Could you check a few things on this model? Use its own coordinates, in mm. A direction names the side the tool comes from. Round coordinates to 2 decimals unless told otherwise and drop trailing zeros. Write each loop counter-clockwise with the first axis right and the second up, starting at its lowest first coordinate (ties: lowest second). Pieces come first, ordered by that corner, then holes. Notation, with made-up numbers: (66.5, 25.25) - (124.5, 25.25) arc R9 cw to (124.5, 38.25) - close; hole circle Ø5 at (61.25, 82). An arc over 180 degrees is marked (long way). Write each question's results on one line, items separated by ' | '. Start each with the question number.
(1) For P1, Ø5, axis at y = 44, z = 7.5, coming from the +X side; P2, Ø3, axis at y = 44, z = 0, coming from the -X side; P3, Ø4, axis at y = -51, z = 10, coming from the -X side, each with a flat end and sliding along its axis, tell me the tip position at first contact or that it passes through.
(2) Thinking about a two-plate mould opening in X: for faces 6 (the flat face through (103, 71.514, 4)), 7 (the cylindrical face through (81.775, 0.208, 5.635)), 8 (the flat face through (101, 35, -0.635)), which applies, +X half, -X half, draft (parallel to the pull), parting line (faces both ways), or undercut?
(3) On a 3-axis mill with a long thin cutter (end or side, diameter ignored), from which of +Z, -Z, +X, -X, +Y, -Y can I reach the whole of each face in a straight line? I mean faces 1 (the flat face through (138.502, 0, 6)), 2 (the cylindrical face through (115.911, 39.965, -1.887)), 3 (the cylindrical face through (119.4, 28.1, 10.2)), 4 (the cylindrical face through (131.746, -52.192, 4.365)), 5 (the cylindrical face through (77.987, 69.223, 4.126)). Say none if no direction works.
(4) Please list where these lines run through material, in increasing order: line 1 (Y direction, x = 93, z = -0.75); line 2 (X direction, y = -5, z = -0.5); line 3 (Y direction, x = 85, z = 6). Write a range as [from, to].
(5) Imagine slicing it at B-B on x = 78.5. Write out the boundary of the cut face in (y, z), then the cut area to 3 significant figures.
(6) Imagine slicing it at C-C on y = -8.5. Write out the boundary of the cut face in (x, z).
(7) Imagine slicing it at A-A on z = 5. Write out the boundary of the cut face in (x, y), then the cut area to 3 significant figures.
```python
from build123d import *

# Parameters (mm, degrees)
SKETCH2_W               = 62.687945492
SKETCH2_H               = 144.612264151
EXTRUDE1_DEPTH          = 11.43
CUT_EXTRUDE2_DEPTH      = 158.024733797
CUT_EXTRUDE2_DEPTH_BACK = 158.024733797
FILLET1_R               = 7.62
CUT_EXTRUDE3_DEPTH      = 158.024733797
CUT_EXTRUDE4_DEPTH      = 11.43
SKETCH6_W               = 12.479780257
SKETCH6_H               = 2.472828988
CUT_EXTRUDE5_DEPTH      = 158.024733797
SKETCH7_R               = 3.81
CUT_EXTRUDE6_DEPTH      = 2.54
EXTRUDE2_DEPTH          = 2.54
SKETCH13_R              = 25
EXTRUDE4_DEPTH          = 0.635
SKETCH14_R              = 21.59
CUT_EXTRUDE7_DEPTH      = 2.54
SKETCH15_R              = 7.62
SKETCH15_R_2            = 5.08
EXTRUDE5_DEPTH          = 2.54
SKETCH16_R              = 2.54
CUT_EXTRUDE8_DEPTH      = 164.951198757
SKETCH17_W              = 37.108426787
SKETCH17_H              = 5.41310776
CUT_EXTRUDE9_DEPTH      = 0.508
SKETCH18_W              = 60.115740974
SKETCH18_H              = 6.745649024
EXTRUDE6_DEPTH          = 0.508


# Read off the part's stored shape, not the designer's step: Cut-Extrude4
with BuildPart() as part:
    # Sketch2 → Extrude1 (new body)
    with BuildSketch(Plane.XY):
        with Locations((107.157914046, -0.792085953)):
            Rectangle(SKETCH2_W, SKETCH2_H)
    extrude(amount=EXTRUDE1_DEPTH)

    # Sketch3 → Cut-Extrude2 (cut, two sides: drawn at the far end of the back side and taken through both)
    with BuildSketch(Plane.XY.offset(11.43).offset(-CUT_EXTRUDE2_DEPTH_BACK)):
        with BuildLine():
            Line((-8.245884216, 283.124432333), (75.8139413, 35.767808979))
            ThreePointArc((75.8139413, 35.767808979), (81.776003849, -0.305809979), (75.8139413, -36.379428938))
            Line((75.8139413, -36.379428938), (-8.245884216, -283.736052291))
            Line((-8.245884216, -283.736052291), (-530.745083766, -283.736052291))
            Line((-530.745083766, -283.736052291), (-530.745083766, 283.124432333))
            Line((-530.745083766, 283.124432333), (-8.245884216, 283.124432333))
        make_face()
    extrude(amount=CUT_EXTRUDE2_DEPTH + CUT_EXTRUDE2_DEPTH_BACK, mode=Mode.SUBTRACT)

    # Fillet1
    fillet1_edges = [part.edges().sort_by_distance(p)[0] for p in [
        (75.8139413, 71.514046122, 5.715),
        (138.501886792, 71.514046122, 5.715),
        (138.501886792, -73.098218029, 5.715),
        (75.8139413, -73.098218029, 5.715),
    ]]
    fillet(fillet1_edges, radius=FILLET1_R)

    # Sketch4 → Cut-Extrude3 (cut, through all)
    with BuildSketch(Plane(origin=(0, 0, 0), x_dir=(0, 0, -1), z_dir=(1, 0, 0))):
        Polygon((-6.9650624, -75.107104489), (-11.43, -36.379428938), (-27.808277113, -36.379428938), (-27.808277113, -75.107104489), align=None)
        Polygon((-6.9650624, 73.913379264), (-11.43, 35.767808979), (-27.808277113, 35.767808979), (-27.808277113, 73.913379264), align=None)
    extrude(amount=CUT_EXTRUDE3_DEPTH, mode=Mode.SUBTRACT)

    # Cut-Extrude4 outline → Cut-Extrude4 (cut)
    with BuildSketch(Plane.XY):
        with BuildLine():
            Line((130.881886792, 71.514046122), (122.168957501, 71.514046122))
            ThreePointArc((122.168957501, 71.514046122), (131.969322241, 51.63307619), (138.501886792, 30.452289734))
            Line((138.501886792, 30.452289734), (138.501886792, 63.894046122))
            ThreePointArc((138.501886792, 63.894046122), (136.270040464, 69.282199795), (130.881886792, 71.514046122))
        make_face()
        with BuildLine():
            Line((138.501886792, -65.478218029), (138.501886792, -30.452289734))
            ThreePointArc((138.501886792, -30.452289734), (131.624319899, -52.492129451), (121.210647413, -73.098218029))
            Line((121.210647413, -73.098218029), (130.881886792, -73.098218029))
            ThreePointArc((130.881886792, -73.098218029), (136.270040465, -70.866371702), (138.501886792, -65.478218029))
        make_face()
    extrude(amount=CUT_EXTRUDE4_DEPTH, mode=Mode.SUBTRACT)

    # Sketch6 → Cut-Extrude5 (cut, through all)
    with BuildSketch(Plane(origin=(0, 0, 0), x_dir=(0, 0, -1), z_dir=(1, 0, 0))):
        with Locations((-15.014254811, -0.20641593)):
            Rectangle(SKETCH6_W, SKETCH6_H)
    extrude(amount=CUT_EXTRUDE5_DEPTH, mode=Mode.SUBTRACT)

    # Sketch7 → Cut-Extrude6 (cut)
    with BuildSketch(Plane.XY.offset(11.43)):
        with Locations((122.168957501, 25.482679021)):
            Circle(SKETCH7_R)
        with Locations((122.168957501, -23.361435355)):
            Circle(SKETCH7_R)
        with Locations((94.197047539, -46.60449668)):
            Circle(SKETCH7_R)
        with Locations((94.197047539, 46.367748617)):
            Circle(SKETCH7_R)
    extrude(amount=-CUT_EXTRUDE6_DEPTH, mode=Mode.SUBTRACT)

    # Sketch11 → Extrude2 (add)
    with BuildSketch(Plane.XY):
        with BuildLine():
            Line((140.459634853, 30.367090459), (140.459634853, -30.772266502))
            ThreePointArc((140.459634853, -30.772266502), (133.081559649, -53.585706853), (122.100984967, -74.900397422))
            Line((122.100984967, -74.900397422), (113.111333503, -74.900397422))
            ThreePointArc((113.111333503, -74.900397422), (111.315282279, -75.644346198), (110.571333503, -77.440397422))
            Line((110.571333503, -77.440397422), (110.571333503, -81.248075827))
            ThreePointArc((110.571333503, -81.248075827), (109.827384728, -83.044127051), (108.031333503, -83.788075827))
            Line((108.031333503, -83.788075827), (96.467437878, -83.788075827))
            ThreePointArc((96.467437878, -83.788075827), (94.671386654, -83.044127051), (93.927437878, -81.248075827))
            Line((93.927437878, -81.248075827), (93.927437878, -77.440397422))
            ThreePointArc((93.927437878, -77.440397422), (93.183489102, -75.644346198), (91.387437878, -74.900397422))
            Line((91.387437878, -74.900397422), (84.20468933, -74.900397422))
            ThreePointArc((84.20468933, -74.900397422), (77.387287325, -72.495127974), (74.267438474, -65.97371445))
            Line((74.267438474, -65.97371445), (74.267438474, -35.993533901))
            ThreePointArc((74.267438474, -35.993533901), (80.424902626, -0.301125715), (74.435866454, 35.419929877))
            Line((74.435866454, 35.419929877), (74.435866454, 65.905394367))
            ThreePointArc((74.435866454, 65.905394367), (76.686596692, 71.178053101), (82.012839907, 73.298866609))
            Line((82.012839907, 73.298866609), (92.429737879, 73.298866609))
            ThreePointArc((92.429737879, 73.298866609), (93.525213934, 74.366945407), (93.927437878, 75.843114776))
            Line((93.927437878, 75.843114776), (93.927437878, 80.272142364))
            ThreePointArc((93.927437878, 80.272142364), (94.671386654, 82.068193588), (96.467437878, 82.812142364))
            Line((96.467437878, 82.812142364), (108.031333503, 82.812142364))
            ThreePointArc((108.031333503, 82.812142364), (109.827384728, 82.068193588), (110.571333503, 80.272142364))
            Line((110.571333503, 80.272142364), (110.571333503, 75.838866609))
            ThreePointArc((110.571333503, 75.838866609), (111.315282279, 74.042815385), (113.111333503, 73.298866609))
            Line((113.111333503, 73.298866609), (122.822960943, 73.298866609))
            ThreePointArc((122.822960943, 73.298866609), (133.212311059, 52.478361728), (140.459634853, 30.367090459))
        make_face()
    extrude(amount=-EXTRUDE2_DEPTH)

    # Sketch13 → Extrude4 (add)
    with BuildSketch(Plane(origin=(202.435743002, 23.123502913, -2.54), x_dir=(-1, 0, 0), z_dir=(0, 0, -1))):
        with Locations((92.140594683, 11.691074744)):
            Circle(SKETCH13_R)
        with Locations((92.140594683, -60.456163173)):
            Circle(SKETCH13_R)
    extrude(amount=EXTRUDE4_DEPTH)

    # Sketch14 → Cut-Extrude7 (cut)
    with BuildSketch(Plane(origin=(0, 0, -3.175), x_dir=(-1, 0, 0), z_dir=(0, 0, -1))):
        with Locations((-110.295148318, 34.814577657)):
            Circle(SKETCH14_R)
        with Locations((-110.295148318, -37.332660261)):
            Circle(SKETCH14_R)
    extrude(amount=-CUT_EXTRUDE7_DEPTH, mode=Mode.SUBTRACT)

    # Sketch15 → Extrude5 (add)
    # profile 1 of 2: a face of its own
    with BuildSketch(Plane(origin=(0, 0, -0.635), x_dir=(-1, 0, 0), z_dir=(0, 0, -1))):
        with Locations((-110.295148318, 34.814577657)):
            Circle(SKETCH15_R)
        with Locations((-110.295148318, 34.814577657)):
            Circle(SKETCH15_R_2, mode=Mode.SUBTRACT)
    # profile 2 of 2: a face of its own
    with BuildSketch(Plane(origin=(0, 0, -0.635), x_dir=(-1, 0, 0), z_dir=(0, 0, -1))):
        with Locations((-110.295148318, -37.332660261)):
            Circle(SKETCH15_R)
        with Locations((-110.295148318, -37.332660261)):
            Circle(SKETCH15_R_2, mode=Mode.SUBTRACT)
    extrude(amount=EXTRUDE5_DEPTH)

    # Sketch16 → Cut-Extrude8 (cut, through all)
    with BuildSketch(Plane.XY):
        with Locations((102.185519341, 77.398921819)):
            Circle(SKETCH16_R)
        with Locations((102.185519341, -79.070725904)):
            Circle(SKETCH16_R)
    extrude(amount=-CUT_EXTRUDE8_DEPTH, mode=Mode.SUBTRACT)

    # Sketch17 → Cut-Extrude9 (cut)
    with BuildSketch(Plane.XY):
        with Locations((105.706841443, -79.117825298)):
            Rectangle(SKETCH17_W, SKETCH17_H)
        with Locations((105.628622382, 77.519388414)):
            Rectangle(SKETCH17_W, SKETCH17_H)
    extrude(amount=-CUT_EXTRUDE9_DEPTH, mode=Mode.SUBTRACT)

    # Sketch18 → Extrude6 (add)
    with BuildSketch(Plane(origin=(0, 0, -2.54), x_dir=(-1, 0, 0), z_dir=(0, 0, -1))):
        with Locations((-110.401764366, -0.863643629)):
            Rectangle(SKETCH18_W, SKETCH18_H)
    extrude(amount=EXTRUDE6_DEPTH)


solid = part.part
```
Response:
1) P1: x = 135.55 | P2: x = 74.44 | P3: x = 75.81
2) face 6: draft | face 7: -X half | face 8: undercut
3) face 1: +Z, +X, +Y, -Y | face 2: -Z | face 3: +Z | face 4: +Z, +X, -Y | face 5: +Z, -X, +Y
4) line 1: [-75.48, -50.26], [-24.41, 21.89], [47.74, 73.71] | line 2: [80.31, 140.46] | line 3: [-73.1, 71.51]
5) outline: (-73.35, -2.54) - (-20.35, -2.54) - (-20.35, 0) - (-27.21, 0) - (-27.21, 11.43) - (-36.38, 11.43) - (-71.29, 7.41) - (-71.29, 0) - (-73.35, 0) - close; (20.26, -2.54) - (72.48, -2.54) - (72.48, 0) - (69.7, 0) - (69.7, 7.46) - (35.77, 11.43) - (26.6, 11.43) - (26.6, 0) - (20.26, 0) - close | area: 1,130 mm²
6) outline: (80.09, -2.54) - (140.46, -2.54) - (140.46, 0) - (138.5, 0) - (138.5, 11.43) - (81.48, 11.43) - (81.48, 0) - (80.09, 0) - close
7) outline: (75.81, -65.48) arc R7.62 ccw to (83.43, -73.1) - (121.21, -73.1) arc R139.7 ccw to (138.5, -30.45) - (138.5, 30.45) arc R139.7 ccw to (122.17, 71.51) - (83.43, 71.51) arc R7.62 ccw to (75.81, 63.89) - (75.81, 35.77) arc R112.11 cw to (75.81, -36.38) - close | area: 8,160 mm²
